Here's how the part is built. I have some questions about the finished solid (model axes, mm). Face numbers are marked on the shaded views. A direction names the side the tool comes from. Coordinates: 2 decimals unless noted, no trailing zeros. Loops run counter-clockwise (first coordinate to the right, second up) from the corner with the lowest first, then second, coordinate; pieces in that order, holes last. Notation, with made-up numbers: M 30,-24.5 L 85,-24.5 A23 ccw 85,-3.5 Z; hole C -6.5,79 d3. An arc over 180 degrees is marked long. Use CSV: the item, a comma, the result in double quotes. Start each with the question number.
Q1. If we section it at A-A (z = 0): Please give me the cut outline in (x, y), and give its area (3 significant figures).
Q2. If we mould it in two halves opening along Y, with no side actions, what happens to the marked faces 1, 2 and 3? For each: +Y half, -Y half, draft (parallel to the pull), parting line (faces both ways), or undercut.
Q3. If we section it at C-C (x = -15): Please give me the cut outline in (y, z).
Q4. Which directions (+Z, -Z, +X, -X, +Y, -Y) give clear straight access to the entire face, cutting with the end or side of a thin tool? Please do the marked faces 4, 5, 6 and 7.
Q5. Please list where these lines run through material, in increasing order: probe 1 along Z at (x, y) = (-0.95, 0); probe 2 along Z at (x, y) = (-17, 0); probe 3 along X at (y, z) = (-7.25, -1.75). Write a range as [from, to].
Q6. For pin 1 Ø4 at (x, y) = (-20, -4) entering from +Z; pin 2 Ø5.5 at (y, z) = (0, 0) entering from -X; pin 3 Ø6 at (y, z) = (-0.5, -1.5) entering from +X, each with a flat end and sliding along its axis, tell me the tip position at first contact or that it passes through.
from build123d import *


with BuildPart() as part:
    # Sketch1 → Revolve1 (revolve)
    with BuildSketch(Plane.XY):
        with BuildLine():
            Line((-2.519270709, 7.706480957), (-1.725734073, 10.668))
            Line((-1.725734073, 10.668), (-0.508, 10.668))
            Line((-0.508, 10.668), (-0.508, 5.842))
            Line((-0.508, 5.842), (-1.4, 5.842))
            Line((-1.4, 5.842), (-1.4, 2.413))
            Line((-1.4, 2.413), (-24.068719082, 2.413))
            Line((-24.068719082, 2.413), (-28.412119082, 6.7564))
            Line((-28.412119082, 6.7564), (-28.412119082, 7.7724))
            Line((-28.412119082, 7.7724), (-15.712119082, 7.7724))
            Line((-15.712119082, 7.7724), (-15.712119082, 10.668))
            Line((-15.712119082, 10.668), (-7.146325468, 10.668))
            Line((-7.146325468, 10.668), (-6.352788832, 7.706480957))
            ThreePointArc((-6.352788832, 7.706480957), (-4.43602977, 6.2357), (-2.519270709, 7.706480957))
        make_face()
    revolve(axis=Axis((-22.598839253, 0, 0), (1, 0, 0)))


solid = part.part
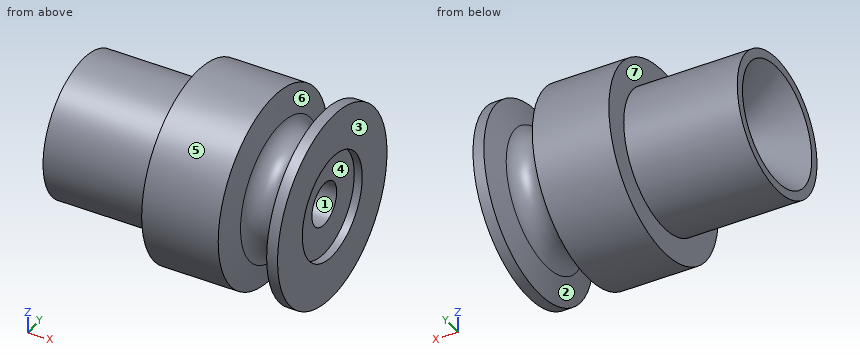
Results below:
1,outline,"M -28.41,-7.77 L -15.71,-7.77 L -15.71,-10.67 L -7.15,-10.67 L -6.35,-7.71 A1.98 cw -2.52,-7.71 L -1.73,-10.67 L -0.51,-10.67 L -0.51,-5.84 L -1.4,-5.84 L -1.4,-2.41 L -24.07,-2.41 L -28.41,-6.76 Z; M -28.41,6.76 L -24.07,2.41 L -1.4,2.41 L -1.4,5.84 L -0.51,5.84 L -0.51,10.67 L -1.73,10.67 L -2.52,7.71 A1.98 cw -6.35,7.71 L -7.15,10.67 L -15.71,10.67 L -15.71,7.77 L -28.41,7.77 Z"
1,area,"326 mm^2"
2,face 1,"undercut"
2,face 2,"parting line"
2,face 3,"draft"
3,outline,"C 0,0 d21.34; hole C 0,0 d4.83"
4,face 4,"+X"
4,face 5,"+X, -X"
4,face 6,"none"
4,face 7,"-X"
5,probe 1,"[-10.67, -5.84], [5.84, 10.67]"
5,probe 2,"[-7.77, -2.41], [2.41, 7.77]"
5,probe 3,"[-28.41, -6.27], [-2.6, -0.51]"
6,pin 1,"z = 7.51"
6,pin 2,"x = -24.41"
6,pin 3,"x = -1.4"
